Source: CAD feature listing. Evaluate the final solid. Frame: model axes, mm. Face numbers are marked on the shaded views. A direction names the side the tool comes from. Round coordinates to 2 decimals unless told otherwise and drop trailing zeros. Write each loop counter-clockwise with the first axis right and the second up, starting at its lowest first coordinate (ties: lowest second). Pieces come first, ordered by that corner, then holes.
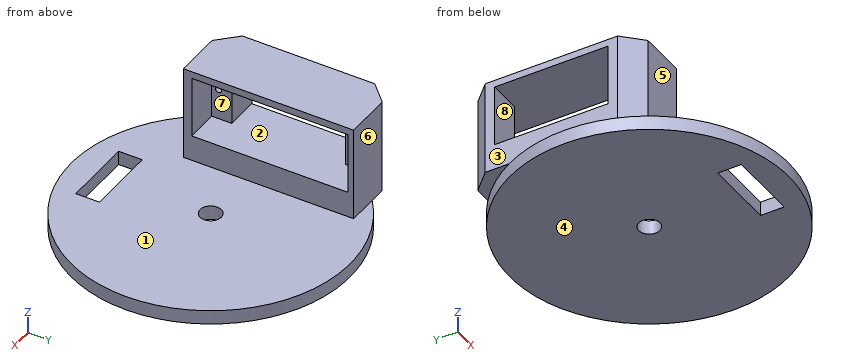
from build123d import *

# Parameters (mm, degrees)
SKETCH046_R     = 29.5
PAD016_DEPTH    = 3
SKETCH047_R     = 2.25
POCKET027_DEPTH = 3
SKETCH048_W     = 15
SKETCH048_H     = 5
POCKET028_DEPTH = 5
SKETCH050_W     = 14
SKETCH050_H     = 36
PAD017_DEPTH    = 20
SKETCH051_W     = 24
SKETCH051_H     = 13
POCKET030_DEPTH = 14
SKETCH052_W     = 33
SKETCH052_H     = 13
POCKET031_DEPTH = 7
SKETCH053_R     = 0.625
POCKET032_DEPTH = 5
CHAMFER001_SIZE = 4


with BuildPart() as part:
    # Sketch046 → Pad016 (new body)
    with BuildSketch(Plane.XY):
        with Locations((0, -11)):
            Circle(SKETCH046_R)
    extrude(amount=PAD016_DEPTH)

    # Sketch047 (on Face2 of Pad016) → Pocket027 (cut)
    with BuildSketch(Plane(origin=(0, 0, 0), x_dir=(1, 0, 0), z_dir=(0, 0, -1))):
        with Locations((0, 11)):
            Circle(SKETCH047_R)
    extrude(amount=-POCKET027_DEPTH, mode=Mode.SUBTRACT)

    # Sketch048 (on Face3 of Pocket027) → Pocket028 (cut)
    with BuildSketch(Plane.XY.offset(3)):
        with Locations((0, -32.5)):
            Rectangle(SKETCH048_W, SKETCH048_H)
    extrude(amount=-POCKET028_DEPTH, mode=Mode.SUBTRACT)

    # Sketch050 (on Face3 of Pocket028) → Pad017 (join)
    with BuildSketch(Plane.XY.offset(3)):
        with Locations((-19, -6)):
            Rectangle(SKETCH050_W, SKETCH050_H)
    extrude(amount=PAD017_DEPTH)

    # Sketch051 (on Face10 of Pad017) → Pocket030 (cut)
    with BuildSketch(Plane(origin=(-26, 0, 0), x_dir=(0, -1, 0), z_dir=(-1, 0, 0))):
        with Locations((6, 15)):
            Rectangle(SKETCH051_W, SKETCH051_H)
    extrude(amount=-POCKET030_DEPTH, mode=Mode.SUBTRACT)

    # Sketch052 (on Face12 of Pocket030) → Pocket031 (cut)
    with BuildSketch(Plane.YZ.offset(-12)):
        with Locations((-5.75, 15)):
            Rectangle(SKETCH052_W, SKETCH052_H)
    extrude(amount=-POCKET031_DEPTH, mode=Mode.SUBTRACT)

    # Sketch053 (on Face27 of Pocket031) → Pocket032 (cut)
    with BuildSketch(Plane.YZ.offset(-19)):
        with Locations((-20.831921, 15)):
            Circle(SKETCH053_R)
        with Locations((9.168079, 15)):
            Circle(SKETCH053_R)
    extrude(amount=-POCKET032_DEPTH, mode=Mode.SUBTRACT)

    # Chamfer001
    chamfer001_edges = [part.edges().sort_by_distance(p)[0] for p in [
        (-26, 12, 13),
        (-26, -24, 13),
    ]]
    chamfer(chamfer001_edges, length=CHAMFER001_SIZE)


with BuildPart() as part_1:
    # Body003 placement: moved
    add(part.part.moved(Location((0, 0, 30))))


solid = part_1.part
1) Pull-direction query (Z, two-part tool) for the marked faces 1, 2, 3 and 4; classes: released by +Z, released by -Z, zero draft, split by the parting line, or undercut.
Taken from the geometry:
face 1: released by +Z
face 2: undercut
face 3: zero draft
face 4: released by -Z
2) Section query C-C on y = 2. Return the cut outline in (x, z), then the cut area to 3 significant figures.
Taken from the geometry:
outline: (-26.48, 30) - (26.48, 30) - (26.48, 33) - (-12, 33) - (-12, 38.5) - (-26, 38.5) - (-26, 33) - (-26.48, 33) - close; (-26, 51.5) - (-12, 51.5) - (-12, 53) - (-26, 53) - close
area: 257 mm2
3) Section query B-B on z = 39.5. Return the cut outline in (x, y), then the cut area to 3 significant figures.
Taken from the geometry:
outline: (-26, -20) - (-22, -24) - (-12, -24) - (-12, -22.25) - (-19, -22.25) - (-19, -18) - (-26, -18) - close; (-26, 6) - (-19, 6) - (-19, 10.75) - (-12, 10.75) - (-12, 12) - (-22, 12) - (-26, 8) - close
area: 89.0 mm2
4) Section query A-A on x = 0. Return the cut outline in (y, z).
Taken from the geometry:
outline: (-40.5, 30) - (-35, 30) - (-35, 33) - (-40.5, 33) - close; (-30, 30) - (-13.25, 30) - (-13.25, 33) - (-30, 33) - close; (-8.75, 30) - (18.5, 30) - (18.5, 33) - (-8.75, 33) - close
5) Material intervals for line 1 (Y direction, x = 0, z = 32.15); line 2 (Y direction, x = -20.6, z = 45); line 3 (Z direction, x = -20.5, y = 3.5), sorted ascending.
Taken from the geometry:
line 1: y = -40.5 to -35, -30 to -13.25, -8.75 to 18.5
line 2: y = -24 to -21.46, -20.21 to -18, 6 to 8.54, 9.79 to 12
line 3: z = 30 to 38.5, 51.5 to 53
6) Reachability of the marked faces 5, 6, 7 and 8 from +Z, -Z, +X, -X, +Y, -Y: full face, straight path, thin tool, end or side. Return the list, or none.
Taken from the geometry:
face 5: +Z, +X, -X, -Y
face 6: +Z, +X, -X, +Y
face 7: +X
face 8: +X, -X
7) Contact query for flat-ended pins moving along their axis: P1, Ø3, axis at x = -16.5, z = 45.5, coming from the -Y side; P2, Ø3, axis at x = -18.5, z = 40.5, coming from the +Y side; P3, Ø1, axis at y = -20.5, z = 45.5, coming from the +X side. Output: stop coordinate, or through.
Taken from the geometry:
P1: stops at y = -24
P2: stops at y = 12
P3: stops at x = -19
8) Section query D-D on x = -15. Return the cut outline in (y, z).
Taken from the geometry:
outline: (-36.4, 30) - (14.4, 30) - (14.4, 33) - (12, 33) - (12, 53) - (-24, 53) - (-24, 33) - (-36.4, 33) - close; hole (-22.25, 38.5) - (10.75, 38.5) - (10.75, 51.5) - (-22.25, 51.5) - close
